```python
from build123d import *

# Parameters (mm, degrees)
SKETCH1_W           = 7.4
SKETCH1_H           = 11.5
BOSS_EXTRUDE1_DEPTH = 11.5
BOSS_EXTRUDE2_DEPTH = 3.1
SKETCH6_W           = 6.05
SKETCH6_H           = 10.1
CUT_EXTRUDE1_DEPTH  = 21.593612692
CUT_EXTRUDE2_DEPTH  = 3.1
SKETCH8_W           = 3
SKETCH8_H           = 3
CUT_EXTRUDE3_DEPTH  = 1.35
CUT_EXTRUDE4_DEPTH  = 1.8
FILLET1_R           = 1
FILLET2_R           = 0.5
FILLET3_R           = 2


# Read off the part's stored shape, not the designer's step: Mirror3
with BuildPart() as part:
    # Sketch1 → Boss-Extrude1 (new body)
    with BuildSketch(Plane(origin=(0, 0, 0), x_dir=(1, 0, 0), z_dir=(0, 1, 0))):
        with Locations((-3.7, 0)):
            Rectangle(SKETCH1_W, SKETCH1_H)
    extrude(amount=BOSS_EXTRUDE1_DEPTH)

    # Sketch3 → Boss-Extrude2 (add)
    with BuildSketch(Plane(origin=(0, 0, 0), x_dir=(1, 0, 0), z_dir=(0, 1, 0))):
        with BuildLine():
            Line((-8.35, 2.749742999), (-7.4, 2.749742999))
            Line((-7.4, 2.749742999), (-7.4, -5.75))
            Line((-7.4, -5.75), (-8.35, -5.75))
            ThreePointArc((-8.35, -5.75), (-12.633049046, -1.500128501), (-8.35, 2.749742999))
        make_face()
    extrude(amount=BOSS_EXTRUDE2_DEPTH)

    # Sketch6 → Cut-Extrude1 (cut, through all)
    with BuildSketch(Plane(origin=(0, 0, -5.75), x_dir=(-1, 0, 0), z_dir=(0, 0, -1))):
        with Locations((3.025, 5.05)):
            Rectangle(SKETCH6_W, SKETCH6_H)
    extrude(amount=-CUT_EXTRUDE1_DEPTH, mode=Mode.SUBTRACT)

    # Sketch7 → Cut-Extrude2 (cut)
    with BuildSketch(Plane.XZ):
        with BuildLine():
            Line((-9.1, 2.600128501), (-6.05, 2.600128501))
            ThreePointArc((-6.05, 2.600128501), (-4.95, 1.500128501), (-6.05, 0.400128501))
            Line((-6.05, 0.400128501), (-9.1, 0.400128501))
            ThreePointArc((-9.1, 0.400128501), (-10.2, 1.500128501), (-9.1, 2.600128501))
        make_face()
    extrude(amount=-CUT_EXTRUDE2_DEPTH, mode=Mode.SUBTRACT)

    # Sketch8 → Cut-Extrude3 (cut)
    with BuildSketch(Plane(origin=(-6.05, 0, 0), x_dir=(0, 0, -1), z_dir=(1, 0, 0))):
        with Locations((-1.500128501, 1.5)):
            Rectangle(SKETCH8_W, SKETCH8_H)
    extrude(amount=-CUT_EXTRUDE3_DEPTH, mode=Mode.SUBTRACT)

    # Sketch9 → Cut-Extrude4 (cut)
    with BuildSketch(Plane(origin=(0, 3.1, 0), x_dir=(1, 0, 0), z_dir=(0, 1, 0))):
        Polygon((-6.85, -2.799166606), (-6.85, -0.201090395), (-9.1, 1.097947711), (-11.35, -0.201090395), (-11.35, -2.799166606), (-9.1, -4.098204712), align=None)
    extrude(amount=-CUT_EXTRUDE4_DEPTH, mode=Mode.SUBTRACT)

    # Fillet1
    # the kernel refuses this fillet: 1 mm, written as the material it adds along each edge
    with BuildSketch(Plane(origin=(-7.4, 3.1, -2.749742999), x_dir=(-1, 0, 0), z_dir=(0, 0, 1))) as fillet1_piece_1_section:
        with BuildLine():
            CenterArc((FILLET1_R, -FILLET1_R), FILLET1_R, 90, 90)
            Line((0, -FILLET1_R), (0, 0))
            Line((0, 0), (FILLET1_R, 0))
        make_face()
    fillet1_piece_1 = extrude(amount=5.133290746, mode=Mode.PRIVATE)
    fillet1_piece_1 = split(fillet1_piece_1, bisect_by=Plane(origin=(-8.63172693, 3.371201356, -0.827590128), z_dir=(0.49999999999999983, 0, -0.8660254037844388)), keep=Keep.TOP, mode=Mode.PRIVATE)
    add(fillet1_piece_1)
    with BuildSketch(Plane(origin=(-7.4, 3.1, -5.249742999), x_dir=(-1, 0, 0), z_dir=(0, 0, 1))) as fillet1_piece_2_section:
        with BuildLine():
            CenterArc((FILLET1_R, -FILLET1_R), FILLET1_R, 90, 90)
            Line((0, -FILLET1_R), (0, 0))
            Line((0, 0), (FILLET1_R, 0))
        make_face()
    fillet1_piece_2 = extrude(amount=7.633290746, mode=Mode.PRIVATE)
    fillet1_piece_2 = fillet1_piece_2 & Plane(origin=(-8.383049046, 3.100281112, 1.500128501), x_dir=(0.007776246012108559, 0, 0.9999697645418881), z_dir=(0, -1, 0)) * Cylinder(4.25, 20, mode=Mode.PRIVATE)
    fillet1_piece_2 = split(fillet1_piece_2, bisect_by=Plane(origin=(-9.26614006, 3.100281112, -1.193868719), z_dir=(0.49999999999999983, 0, -0.8660254037844388)), keep=Keep.TOP, mode=Mode.PRIVATE)
    add(fillet1_piece_2)
    with BuildSketch(Plane(origin=(-7.4, 3.1, 0.616709254), x_dir=(-1, 0, 0), z_dir=(0, 0, 1))) as fillet1_piece_3_section:
        with BuildLine():
            CenterArc((FILLET1_R, -FILLET1_R), FILLET1_R, 90, 90)
            Line((0, -FILLET1_R), (0, 0))
            Line((0, 0), (FILLET1_R, 0))
        make_face()
    fillet1_piece_3 = extrude(amount=5.133290746, mode=Mode.PRIVATE)
    fillet1_piece_3 = split(fillet1_piece_3, bisect_by=Plane(origin=(-8.144343012, 3.326849972, 3.546455893), z_dir=(0.5000000000000008, 0, 0.8660254037844383)), keep=Keep.TOP, mode=Mode.PRIVATE)
    add(fillet1_piece_3)
    with BuildSketch(Plane(origin=(-7.4, 3.1, 0.616709254), x_dir=(-1, 0, 0), z_dir=(0, 0, 1))) as fillet1_piece_4_section:
        with BuildLine():
            CenterArc((FILLET1_R, -FILLET1_R), FILLET1_R, 90, 90)
            Line((0, -FILLET1_R), (0, 0))
            Line((0, 0), (FILLET1_R, 0))
        make_face()
    fillet1_piece_4 = extrude(amount=7.633290746, mode=Mode.PRIVATE)
    fillet1_piece_4 = fillet1_piece_4 & Plane(origin=(-8.383049046, 3.100281111, 1.500128501), x_dir=(0.007776246012108559, 0, 0.9999697645418881), z_dir=(0, -1, 0)) * Cylinder(4.25, 20, mode=Mode.PRIVATE)
    fillet1_piece_4 = split(fillet1_piece_4, bisect_by=Plane(origin=(-9.266139995, 3.100281111, 4.194125683), z_dir=(0.5000000000000008, 0, 0.8660254037844383)), keep=Keep.TOP, mode=Mode.PRIVATE)
    add(fillet1_piece_4)

    # Fillet2
    fillet2_edges = [part.edges().sort_by_distance(p)[0] for p in [
        (-7.4, 11.5, 0),
    ]]
    fillet(fillet2_edges, radius=FILLET2_R)

    # Fillet3
    fillet3_edges = [part.edges().sort_by_distance(p)[0] for p in [
        (-6.05, 10.1, 0),
    ]]
    fillet(fillet3_edges, radius=FILLET3_R)

    # Mirror3: part across plane


with BuildPart() as part_1:
    add(part.part)
    add(part.part.mirror(Plane(origin=(0, 0, 0), x_dir=(0, 0, 1), z_dir=(1, 0, 0))))


solid = part_1.part
```
Check sheet for the modelled part. Datum: model origin and axes. Units: mm. A direction names the side the tool comes from. Give positions to 0.01 mm unless a question says otherwise; leave off trailing zeros. Write each loop counter-clockwise with the first axis right and the second up, starting at its lowest first coordinate (ties: lowest second). Pieces come first, ordered by that corner, then holes. Notation, with made-up numbers: (-8.5, 5.25) - (7.5, 5.25) arc R9 cw to (7.5, 17.25) - close; hole circle Ø3 at (14, 88). An arc over 180 degrees is marked (long way). Answer as a JSON object with one key per item and string values. Group by question number.
1) Sectioned sample at D-D (z = -5). Record the cut outline in (x, y), then the cut area to 3 significant figures.
2) Sectioned sample at B-B (x = -8). Record the cut outline in (y, z), then the cut area to 3 significant figures.
3) Depth check by flat-ended pin: P1, Ø1, axis at x = -8, z = 3, coming from the -Y side; P2, Ø3, axis at y = 10, z = -2, coming from the -X side; P3, Ø0.7, axis at x = 6.5, z = 2, coming from the -Y side; P4, Ø1.5, axis at x = 0.5, z = 3, coming from the -Y side. Enter the tip coordinate at first touch or a pass-through.
4) Sectioned sample at A-A (y = 7.75). Record the cut outline in (x, z), then the cut area to 4 significant figures.
5) Thickness scan on probe 1 along X at (y, z) = (3.5, -4.5); probe 2 along Y at (x, z) = (10.25, -2). Record the ranges inside material, lowest first. Write a range as from..to.
6) Sectioned sample at C-C (z = 1). Record the cut outline in (x, y), then the cut area to 3 significant figures.
7) Access from +Z, -Z, +X, -X, +Y, -Y to the whole of each face (thin tool, end or side, straight path). Record for faces 1 (the face through (12, 3.1, 1)), 2 (the face through (10.209, 2.213, -0.458)), 3 (the face through (10.2, 0.6, 1.5)), 4 (the face through (0, 10.1, 0)).
Geometry results:
{
 "1": {"outline": "(-7.4, 0) - (-6.05, 0) - (-6.05, 8.1) arc R2 cw to (-4.05, 10.1) - (4.05, 10.1) arc R2 cw to (6.05, 8.1) - (6.05, 0) - (7.4, 0) - (7.4, 11) arc R0.5 ccw to (6.9, 11.5) - (-6.9, 11.5) arc R0.5 ccw to (-7.4, 11) - close", "area": "49.6 mm^2"},
 "2": {"outline": "(0, -2.75) - (3.18, -2.75) - (3.18, -0.46) - (1.3, -0.46) - (1.3, 0.4) - (0, 0.4) - close; (0, 2.6) - (1.3, 2.6) - (1.3, 3.46) - (3.18, 3.46) - (3.18, 5.75) - (0, 5.75) - close", "area": "16.8 mm^2"},
 "3": {"P1": "stops at y = 0", "P2": "stops at x = -7.4", "P3": "stops at y = 3.1", "P4": "stops at y = 10.1"},
 "4": {"outline": "(-7.4, -5.75) - (-6.05, -5.75) - (-6.05, 5.75) - (-7.4, 5.75) - close; (6.05, -5.75) - (7.4, -5.75) - (7.4, 5.75) - (6.05, 5.75) - close", "area": "31.05 mm^2"},
 "5": {"probe 1": "x = -7.4..-6.05, 6.05..7.4", "probe 2": "y = 0..3.1"},
 "6": {"outline": "(-12.6, 0) - (-10.08, 0) - (-10.08, 1.3) - (-11.35, 1.3) - (-11.35, 3.1) - (-12.6, 3.1) - close; (-7.4, 3.1) - (-6.05, 3.1) - (-6.05, 8.1) arc R2 cw to (-4.05, 10.1) - (4.05, 10.1) arc R2 cw to (6.05, 8.1) - (6.05, 3.1) - (7.4, 3.1) - (7.4, 11) arc R0.5 ccw to (6.9, 11.5) - (-6.9, 11.5) arc R0.5 ccw to (-7.4, 11) - close; (10.08, 0) - (12.6, 0) - (12.6, 3.1) - (11.35, 3.1) - (11.35, 1.3) - (10.08, 1.3) - close", "area": "52.3 mm^2"},
 "7": {"face 1": "+Z, -Z, +X, +Y", "face 2": "+Y", "face 3": "+Y, -Y", "face 4": "+Z, -Z, -Y"}
}
